Build history of the part. All positions in model axes, mm. A direction names the side the tool comes from. Give positions to 0.01 mm unless a question says otherwise; leave off trailing zeros. Loops run counter-clockwise (first coordinate to the right, second up) from the corner with the lowest first, then second, coordinate; pieces in that order, holes last. Notation, with made-up numbers: M -11.75,2.5 L 25.25,2.5 A18 cw 25.25,33.5 Z; hole C 18.5,81 d10. An arc over 180 degrees is marked long. Answer as a JSON object with one key per item and string values. Group by question number.
1. Slice it at D-D (y = 32.5). List the corners of the cut face in (x, z), then the cut area to 3 significant figures.
2. Drill centre lines: line 1 along Y through (x, z) = (-2.85, 1.5); line 2 along Y through (x, z) = (-84.05, 1.6); line 3 along Z through (x, y) = (-14, 30). Where is each one in solid material? Low to high. Write a range as [from, to].
3. Slice it at A-A (x = -84.05). List the corners of the cut face in (y, z), then the cut area to 3 significant figures.
4. Slice it at C-C (z = 9.75). List the corners of the cut face in (x, y), then the cut area to 3 significant figures.
5. Drop flat-ended pins along their axis: pin 1 Ø10 at (x, z) = (-22, 17.5) entering from +Y; pin 2 Ø4 at (x, y) = (-55.5, 8) entering from +Z; pin 3 Ø6 at (y, z) = (30, 12) entering from +X; pin 4 Ø2 at (x, y) = (-84.05, 84.05) entering from +Z. Give the stop position or say it passes through.
6. Mould opens along Z. For faces 1 (the face through (-51, 58.32, 11)), 2 (the face through (-3.5, 43, 10)), 3 (the face through (-44, 7, 2)) say: released by +Z, released by -Z, zero draft, split by the parting line, or undercut.
7. 3-axis set-ups, long thin cutter, end or side, ignore diameter. For faces 4 (the face through (-80.95, 85, 1)), 5 (the face through (-51, 37, 18.8)), 6 (the face through (-44, 73, 2)): which of +Z, -Z, +X, -X, +Y, -Y reach the whole face in a straight line?
8. Slice it at B-B (x = -40.5). List the corners of the cut face in (y, z), then the cut area to 3 significant figures.
from build123d import *

# Parameters (mm, degrees)
SKETCH1_W               = 86.9
SKETCH1_H               = 86.9
BOSS_EXTRUDE1_DEPTH     = 2
SKETCH2_R               = 1.65
CUT_EXTRUDE3_DEPTH      = 123.911431527
SKETCH5_W               = 86.9
SKETCH5_H               = 47
BOSS_EXTRUDE3_DEPTH     = 18.8
CUT_EXTRUDE5_START      = -2
SKETCH6_W               = 73.78
SKETCH6_H               = 16.8
CUT_EXTRUDE5_DEPTH      = 43
CUT_EXTRUDE7_DEPTH      = 125.324816509
CUT_EXTRUDE7_DEPTH_BACK = 125.324816509
SKETCH8_W               = 3.5
SKETCH8_H               = 75
SKETCH8_W_2             = 75
SKETCH8_H_2             = 3.5


with BuildPart() as part:
    # Sketch1 → Boss-Extrude1 (new body)
    with BuildSketch(Plane(origin=(0, 0, 0), x_dir=(0, 1, 0), z_dir=(0, 0, 1))):
        with Locations((43.45, 43.45)):
            Rectangle(SKETCH1_W, SKETCH1_H)
    extrude(amount=BOSS_EXTRUDE1_DEPTH)

    # Sketch2 → Cut-Extrude3 (cut, through all)
    with BuildSketch(Plane.XY.offset(2)):
        with Locations((-84.05, 2.85)):
            Circle(SKETCH2_R)
        with Locations((-2.85, 2.85)):
            Circle(SKETCH2_R)
        with Locations((-2.85, 84.05)):
            Circle(SKETCH2_R)
        with Locations((-84.05, 84.05)):
            Circle(SKETCH2_R)
    extrude(amount=-CUT_EXTRUDE3_DEPTH, mode=Mode.SUBTRACT)

    # Sketch5 → Boss-Extrude3 (add)
    with BuildSketch(Plane.XY.offset(2)):
        with Locations((-43.45, 36.82)):
            Rectangle(SKETCH5_W, SKETCH5_H)
    extrude(amount=BOSS_EXTRUDE3_DEPTH)

    # Sketch6 → Cut-Extrude5 (cut)
    with BuildSketch(Plane.XZ.offset(-13.32).offset(CUT_EXTRUDE5_START)):
        with Locations((-50.01, 10.4)):
            Rectangle(SKETCH6_W, SKETCH6_H)
    extrude(amount=-CUT_EXTRUDE5_DEPTH, mode=Mode.SUBTRACT)

    # Sketch8 → Cut-Extrude7 (cut, two sides: drawn at the far end of the back side and taken through both)
    with BuildSketch(Plane.XY.offset(2).offset(-CUT_EXTRUDE7_DEPTH_BACK)):
        with Locations((-1.75, 43.45)):
            Rectangle(SKETCH8_W, SKETCH8_H)
        with Locations((-43.45, 85.15)):
            Rectangle(SKETCH8_W_2, SKETCH8_H_2)
    extrude(amount=CUT_EXTRUDE7_DEPTH + CUT_EXTRUDE7_DEPTH_BACK, mode=Mode.SUBTRACT)


solid = part.part
Established:
{
 "1": {"outline": "M -86.9,0 L -3.5,0 L -3.5,20.8 L -86.9,20.8 L -86.9,18.8 L -13.12,18.8 L -13.12,2 L -86.9,2 Z", "area": "495 mm^2"},
 "2": {"line 1": "y = [0, 1.2], [4.5, 5.95], [80.95, 82.4], [85.7, 86.9]", "line 2": "y = [0, 1.2], [4.5, 82.4], [85.7, 86.9]", "line 3": "z = [0, 2], [18.8, 20.8]"},
 "3": {"outline": "M 0,0 L 1.2,0 L 1.2,2 L 0,2 Z; M 4.5,0 L 82.4,0 L 82.4,2 L 60.32,2 L 60.32,20.8 L 13.32,20.8 L 13.32,2 L 4.5,2 Z; M 85.7,0 L 86.9,0 L 86.9,2 L 85.7,2 Z; hole M 15.32,2 L 58.32,2 L 58.32,18.8 L 15.32,18.8 Z", "area": "322 mm^2"},
 "4": {"outline": "M -86.9,13.32 L -3.5,13.32 L -3.5,60.32 L -86.9,60.32 L -86.9,58.32 L -13.12,58.32 L -13.12,15.32 L -86.9,15.32 Z", "area": "747 mm^2"},
 "5": {"pin 1": "stops at y = 60.32", "pin 2": "stops at z = 2", "pin 3": "stops at x = -3.5", "pin 4": "passes through"},
 "6": {"face 1": "undercut", "face 2": "zero draft", "face 3": "released by +Z"},
 "7": {"face 4": "+Z, -Z, +Y", "face 5": "-X", "face 6": "+Z, +X, -X, +Y"},
 "8": {"outline": "M 0,0 L 83.4,0 L 83.4,2 L 60.32,2 L 60.32,20.8 L 13.32,20.8 L 13.32,2 L 0,2 Z; hole M 15.32,2 L 58.32,2 L 58.32,18.8 L 15.32,18.8 Z", "area": "328 mm^2"}
}
